Autodesk Inventor part; units mm, degrees
ref_plane "YZ Plane" through (0, 0, 0) normal (1, 0, 0) x (0, 1, 0)
ref_plane "XZ Plane" through (0, 0, 0) normal (0, 1, 0) x (-1, 0, 0)
ref_plane "XY Plane" through (0, 0, 0) normal (0, 0, 1) x (1, 0, 0)
ref_plane "Work Plane1" through (0, 0, 0) normal (0, 0, 1) x (1, 0, 0)
sketch "Sketch1" plane through (0, 0, 0) normal (0, 0, 1) x (1, 0, 0)
  circle A0 centre (-28.8, -46.8) radius 1.6
  line L0 (-27.8762, -45.2) -> (-26.9525, -46.8)
  line L1 (-26.9525, -46.8) -> (-27.8762, -48.4)
  line L2 (-27.8762, -48.4) -> (-29.7238, -48.4)
  line L3 (-29.7238, -48.4) -> (-30.6475, -46.8)
  line L4 (-30.6475, -46.8) -> (-29.7238, -45.2)
  line L5 (-29.7238, -45.2) -> (-27.8762, -45.2)
  point P0 (0, 0)
  point P1 (-28.8, -45.2)
extrude "Extrusion1" add sketch "Sketch1" along normal blind 16.5
sketch "Sketch2" plane through (0, 0, 0) normal (0, 0, -1) x (-1, 0, 0)
  circle A0 centre (28.8, -46.8) radius 1.5
  point P0 (0, 0)
  dimension "d2" = 3
extrude "Extrusion2" add sketch "Sketch2" along normal blind 6
properties part number "nanopc_t4_spacer_long" material "Brass, Soft Yellow"
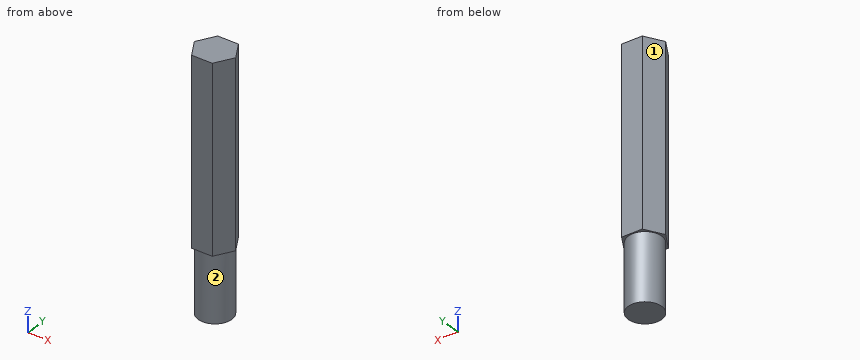
CAD build for the part. Positions are in the model's coordinates, mm. Face numbers are marked on the shaded views. A direction names the side the tool comes from. Coordinates: 2 decimals unless noted, no trailing zeros. Order: outer loops, then holes, each group sorted by start corner. A loop starts at its lowest first (then second) coordinate and runs counter-clockwise, first axis right, second up. Notation, with made-up numbers: M -26,56.5 L -11,56.5 A21 ccw -11,87.5 Z; hole C -29,59 d4. An arc over 180 degrees is marked long. Answer as CSV lines item,"result".
1) 3-axis set-ups, long thin cutter, end or side, ignore diameter. For the marked faces 1 and 2: which of +Z, -Z, +X, -X, +Y, -Y reach the whole face in a straight line?
Verdict:
face 1,"+Z, -Z, -X, +Y"
face 2,"-Z"
2) Drill centre lines: L1, parallel to X at y = -47.6, z = 9.5; L2, parallel to X at y = -47.25, z = 5; L3, parallel to Y at x = -27.65, z = 8.75. Where is each one in solid material? Low to high. Write a range as from..to.
Verdict:
L1,"-30.19..-27.41"
L2,"-30.39..-27.21"
L3,"-48.01..-45.59"
3) Cut at B-B (y = -47.9). List the corners of the cut face in (x, z), then the cut area to 3 significant figures.
Verdict:
outline,"M -30.01,0 L -29.82,0 L -29.82,-6 L -27.78,-6 L -27.78,0 L -27.59,0 L -27.59,16.5 L -30.01,16.5 Z"
area,"52.2 mm2"
4) Cut at A-A (x = -28.8). List the corners of the cut face in (y, z).
Verdict:
outline,"M -48.4,0 L -48.3,0 L -48.3,-6 L -45.3,-6 L -45.3,0 L -45.2,0 L -45.2,16.5 L -48.4,16.5 Z"
5) Cut at C-C (z = -1.5). List the corners of the cut face in (x, y), then the cut area to 3 significant figures.
Verdict:
outline,"C -28.8,-46.8 d3"
area,"7.07 mm2"
6) Flat gauge pin, fed straight in: P1, Ø1, axis at x = -28, z = -3, coming from the +Y side. Where does the tip first touch, or does it go through?
Verdict:
P1,"y = -45.33"
7) Cut at D-D (z = 8.5). List the corners of the cut face in (x, y).
Verdict:
outline,"M -30.65,-46.8 L -29.72,-48.4 L -27.88,-48.4 L -26.95,-46.8 L -27.88,-45.2 L -29.72,-45.2 Z"
